Part model, mm, in its own coordinate system. A direction names the side the tool comes from. Round coordinates to 2 decimals unless told otherwise and drop trailing zeros. Order: outer loops, then holes, each group sorted by start corner. A loop starts at its lowest first (then second) coordinate and runs counter-clockwise, first axis right, second up. Notation, with made-up numbers: (-36.75, 89) -> (4.25, 89) arc R11 cw to (4.25, 110) -> close; hole circle Ø9 at (-1, -7). An arc over 180 degrees is marked (long way). Answer as a JSON object with one key per item and string values. Group by question number.
Autodesk Inventor part; units mm, degrees
ref_plane "Work Plane1" through (0, 0, -34) normal (0, 0, 1) x (1, 0, 0)
ref_plane "YZ Plane" through (0, 0, 0) normal (1, 0, 0) x (0, 1, 0)
ref_plane "XZ Plane" through (0, 0, 0) normal (0, 1, 0) x (-1, 0, 0)
sketch "Sketch1" plane through (0, 0, 0) normal (0, 0, 1) x (1, 0, 0)
  circle A0 centre (0, 0) radius 10
  circle A1 centre (0, 0) radius 17.5
  line L0 (-3, 9.5394) -> (-3, 12)
  line L1 (-3, 12) -> (3, 12)
  line L2 (3, 12) -> (3, 9.5394)
  line L3 (-8.124, -15.5) -> (8.124, -15.5)
  dimension "d0" = 20
  dimension "d1" = 35
  dimension "d2" = 12
  dimension "d3" = 6
  dimension "d4" = 15.5
extrude "Extrusion1" add sketch "Sketch1" along normal mid plane 40 contours A0 | A0 L0 L1 L2 | A1 L3 | L3 A1
extrude "Extrusion2" [suppressed]
chamfer "Chamfer1" [suppressed]
sketch "Sketch2" plane through (0, 0, 0) normal (0, 1, 0) x (-1, 0, 0)
  line L0 (0, 10) -> (0, -10)
  point P0 (0, 0)
  point P1 (0, 0)
  dimension "d12" = 20
hole "Hole1" [suppressed]
sketch "Sketch3" plane through (0, 0, -20) normal (0, 0, -1) x (-1, 0, 0)
  circle A0 centre (0, 0) radius 17.5
  circle A1 centre (0, 0) radius 62.5
  circle A2 centre (0, 0) radius 20
  circle A3 centre (0, 0) radius 56.5
  dimension "d32" = 125
  dimension "d45" = 6
  dimension "d46" = 40
extrude "Extrusion3" add sketch "Sketch3" along normal blind 28 contours A0 | A1 | A2 | A3
ref_plane "Work Plane1" through (0, 0, -34) normal (0, 0, 1) x (1, 0, 0)
extrude "Extrusion4" cut sketch "Sketch3" along normal blind 3.5 contours A3
mirror "Mirror1" about plane through (0, 0, -34) normal (0, 0, 1) of "Extrusion4"
sketch "Sketch4" plane through (0, 0, -48) normal (0, 0, -1) x (-1, 0, 0)
  point P0 (0, 0)
  point P1 (0, 0)
  point P2 (0, 0)
hole "Hole2" at (0, 0, -48) direction (0, 0, 1) diameter 6.6 end through all counterbore diameter 11 counterbore depth 20
chamfer "Chamfer2" distance 1.75 angle 45 1 edges at (-17.5, 0, 20)
sketch "Sketch5" plane through (0, 0, 0) normal (1, 0, 0) x (0, 1, 0)
  line L0 (62.5, -23.137) -> (51.5, -26.5)
  line L1 (51.5, -26.5) -> (51.5, -29.5)
  line L2 (51.5, -29.5) -> (62.5, -32.863)
  line L3 (51.5, -28) -> (62.5, -28) construction
  line L4 (62.5, -23.137) -> (62.5, -32.863)
  line L5 (62.5, -20) -> (62.5, -48)
  line L6 (0, -57.6) -> (0, 9.6)
  point P0 (0, 0)
  dimension "d34" = 34
  dimension "d35" = 11
  dimension "d39" = 3
  dimension "d40" = 8
revolve "Revolution1" cut sketch "Sketch5" angle 360 about axis through (0, 0, -10) along (0, 0, 1)
pattern_linear "Rectangular Pattern1" count 2 spacing 12 along (0, 0, -1) of "Revolution1"
extrude "Extrusion5" cut sketch "Sketch1" along normal through all contours A0 | A0 L0 L1 L2
chamfer "Chamfer3" distance 1.75 angle 45 1 edges at (0, -5.5, -48)
equation "\"d34\" = d37"
equation "\"d35\" = d38"
equation "\"d36\" = 8.5"
equation "\"d37\" = 34deg"
equation "\"d38\" = 11"
properties part number "PWTR-0094" material "Stainless Steel"
Q1. Band-saw the part on A-A (z = -14.5). List the corners of the cut face in (x, y).
Q2. Two-plate mould, pull along Z, no slides. Class faces 5 (the cylindrical face through (5.37, -1.19, -37)), 6 (the cylindrical face through (-50.275, -11.164, -40.021)), 7 (the flat face through (47, -32, -48)): +Z half, -Z half, draft (parallel to the pull), parting line (faces both ways), or undercut.
Q3. Drop flat-ended pins along their axis: pin 1 Ø9 at (x, y) = (2, -1.5) entering from -Z; pin 2 Ø0.7 at (y, z) = (11, 13) entering from +X; pin 3 Ø8 at (x, z) = (-17.5, 13) entering from +Y; pin 4 Ø6 at (x, y) = (0, 0) entering from -Z. Give the stop position or say it passes through.
Q4. Wall check: line 1 (Y direction, x = 0, z = -45.45); line 2 (Z direction, x = -13, y = 52); line 3 (Z direction, x = 2, y = 52.5). Give the ranges that are in metal, low to high. Write a range as [from, to].
Q5. Which spindle directions (+Z, -Z, +X, -X, +Y, -Y) get a long thin tool onto all of the face, cutting with end or side? Do faces 1 (the cylindrical face through (-2.23, -2.43, -13.8)), 2 (the flat face through (0, 12, 10)), 3 (the cylindrical face through (-50.275, -11.164, -28.021)), 4 (the cylindrical face through (4.336, -19.524, -46.274)). Say none if no direction does.
Completed:
{
 "1": {"outline": "circle Ø35 at (0, 0); hole circle Ø6.6 at (0, 0)"},
 "2": {"face 5": "draft", "face 6": "undercut", "face 7": "-Z half"},
 "3": {"pin 1": "z = -47.75", "pin 2": "x = 13.89", "pin 3": "y = 11.14", "pin 4": "through"},
 "4": {"line 1": "[-62.5, -56.5], [-20, -5.5], [5.5, 20], [56.5, 62.5]", "line 2": "[-44.5, -42.14], [-37.86, -30.14], [-25.86, -23.5]", "line 3": "[-44.5, -41.82], [-38.18, -29.82], [-26.18, -23.5]"},
 "5": {"face 1": "+Z, -Z", "face 2": "+Z", "face 3": "none", "face 4": "-Z"}
}
